Here's how the part is built. I have some questions about the finished solid (model axes, mm). Give positions to 0.01 mm unless a question says otherwise; leave off trailing zeros. Write each loop counter-clockwise with the first axis right and the second up, starting at its lowest first coordinate (ties: lowest second). Pieces come first, ordered by that corner, then holes. Notation, with made-up numbers: (63, -29) -> (94, -29) arc R14 cw to (94, -21) -> close; hole circle Ø9 at (71.25, -35.75). An arc over 180 degrees is marked (long way). Use CSV: the item, a comma, the result in double quotes. Start each with the question number.
(1) Suppose I cut it at B-B on x = -6.9. List the corners of the cut face in (y, z) for me.
(2) Suppose I cut it at A-A on z = -5.25. List the corners of the cut face in (x, y) for me, plus the area to 3 significant figures.
(3) Suppose I cut it at C-C on y = 0.55. List the corners of the cut face in (x, z) for me, plus the area to 3 significant figures.
(4) If we mould it in two halves opening along Z, with no side actions, what happens to faces 1 (the flat face through (0, 1, -11)), 2 (the flat face through (0, 0, 0)), 3 (the flat face through (0, 1, 11)), 4 (the cylindrical face through (6.77, 0.99, -4.26))? For each: pulls with the +Z half, pulls with the -Z half, needs draft (parallel to the pull), parting line crosses it, or undercut.
(5) I need wall thicknesses on L1, parallel to Z at x = 6.9, y = 1.4; L2, parallel to X at y = 0.7, z = 5.25; L3, parallel to X at y = 0.7, z = 5.75. Which ranges of each line are inside material? Lowest first, please. Write a range as [from, to].
(6) For pin 1 Ø6 at (x, z) = (1.5, -6.5) entering from -Y; pin 2 Ø1.8 at (x, z) = (6.9, 5.25) entering from +Y, each with a flat end and sliding along its axis, tell me the tip position at first contact or that it passes through.
from build123d import *

# Parameters (mm, degrees)
SKETCH1_W           = 29.8
SKETCH1_H           = 22
BOSS_EXTRUDE1_DEPTH = 2
SKETCH2_R           = 1
CUT_EXTRUDE2_DEPTH  = 10


with BuildPart() as part:
    # Sketch1 → Boss-Extrude1 (new body)
    with BuildSketch(Plane(origin=(0, 0, 0), x_dir=(1, 0, 0), z_dir=(0, 1, 0))):
        Rectangle(SKETCH1_W, SKETCH1_H)
    extrude(amount=BOSS_EXTRUDE1_DEPTH)

    # Sketch2 → Cut-Extrude2 (cut)
    with BuildSketch(Plane.XZ):
        with Locations((6.9, -5.25)):
            Circle(SKETCH2_R)
        with Locations((-6.9, -5.25)):
            Circle(SKETCH2_R)
    cut_extrude2 = extrude(amount=-CUT_EXTRUDE2_DEPTH, mode=Mode.SUBTRACT)

    # Mirror1: Cut-Extrude2 across plane
    add(cut_extrude2.mirror(Plane(origin=(0, 0, 0), x_dir=(1, 0, 0), z_dir=(0, 0, -1))), mode=Mode.SUBTRACT)


solid = part.part
Geometry says:
1,outline,"(0, -11) -> (2, -11) -> (2, -6.25) -> (0, -6.25) -> close; (0, -4.25) -> (2, -4.25) -> (2, 4.25) -> (0, 4.25) -> close; (0, 6.25) -> (2, 6.25) -> (2, 11) -> (0, 11) -> close"
2,outline,"(-14.9, 0) -> (-7.9, 0) -> (-7.9, 2) -> (-14.9, 2) -> close; (-5.9, 0) -> (5.9, 0) -> (5.9, 2) -> (-5.9, 2) -> close; (7.9, 0) -> (14.9, 0) -> (14.9, 2) -> (7.9, 2) -> close"
2,area,"51.6 mm²"
3,outline,"(-14.9, -11) -> (14.9, -11) -> (14.9, 11) -> (-14.9, 11) -> close; hole circle Ø2 at (-6.9, -5.25); hole circle Ø2 at (-6.9, 5.25); hole circle Ø2 at (6.9, -5.25); hole circle Ø2 at (6.9, 5.25)"
3,area,"643 mm²"
4,face 1,"pulls with the -Z half"
4,face 2,"needs draft"
4,face 3,"pulls with the +Z half"
4,face 4,"undercut"
5,L1,"[-11, -6.25], [-4.25, 4.25], [6.25, 11]"
5,L2,"[-14.9, -7.9], [-5.9, 5.9], [7.9, 14.9]"
5,L3,"[-14.9, -7.77], [-6.03, 6.03], [7.77, 14.9]"
6,pin 1,"y = 0"
6,pin 2,"through"
